Geometry: final body of the model. Coordinates: model frame, mm. A direction names the side the tool comes from. Give positions to 0.01 mm unless a question says otherwise; leave off trailing zeros. Write each loop counter-clockwise with the first axis right and the second up, starting at its lowest first coordinate (ties: lowest second). Pieces come first, ordered by that corner, then holes. Notation, with made-up numbers: M 41,27.5 L 48,27.5 A22 cw 48,66.5 Z; hole C 75,1.5 d9. An arc over 180 degrees is marked long. Answer as a JSON object with one key per item and string values.
from build123d import *

# Parameters (mm, degrees)
F0_R          = 342.9
F0_R_2        = 303.53
F1_DEPTH      = 91.44
F1_DEPTH_BACK = 36
F2_R          = 307.34
F2_R_2        = 303.53
F3_DEPTH      = 60.96
F4_R          = 307.34
F4_R_2        = 303.53
F5_DEPTH      = 24


with BuildPart() as f1:
    # F0 (on Front) → F1 (new body, two sides)
    with BuildSketch(Plane.XZ) as f1_sk:
        Circle(F0_R)
        Circle(F0_R_2, mode=Mode.SUBTRACT)
    extrude(amount=F1_DEPTH)
    extrude(f1_sk.sketch, amount=-F1_DEPTH_BACK)

    # F2 (on face) → F3 (cut)
    with BuildSketch(Plane.XZ.offset(91.44)):
        Circle(F2_R)
        Circle(F2_R_2, mode=Mode.SUBTRACT)
    extrude(amount=-F3_DEPTH, mode=Mode.SUBTRACT)

    # F4 (on face) → F5 (cut)
    with BuildSketch(Plane(origin=(0, 36, 0), x_dir=(-1, 0, 0), z_dir=(0, 1, 0))):
        Circle(F4_R)
        Circle(F4_R_2, mode=Mode.SUBTRACT)
    extrude(amount=-F5_DEPTH, mode=Mode.SUBTRACT)


solid = f1.part
1) Cut plane C-C on y = -42. Return loops of the section in (x, z).
Geometry check:
{"outline": "C 0,0 d685.8; hole C 0,0 d614.68"}
2) Cut plane A-A on x = 0. Return loops of the section in (y, z), and give its area (3 significant figures).
Geometry check:
{"outline": "M -91.44,-342.9 L 36,-342.9 L 36,-307.34 L 12,-307.34 L 12,-303.53 L -30.48,-303.53 L -30.48,-307.34 L -91.44,-307.34 Z; M -91.44,307.34 L -30.48,307.34 L -30.48,303.53 L 12,303.53 L 12,307.34 L 36,307.34 L 36,342.9 L -91.44,342.9 Z", "area": "9,390 mm2"}
3) Line query: line 1 (Z direction, x = 0, y = -54); line 2 (Z direction, x = 0, y = -2); line 3 (Z direction, x = -312, y = -42). Output: solid intervals per line, ascending. Write a range as from..to.
Geometry check:
{"line 1": "z = -342.9..-307.34, 307.34..342.9", "line 2": "z = -342.9..-303.53, 303.53..342.9", "line 3": "z = -142.25..142.25"}
4) Contact query for flat-ended pins moving along their axis: P1, Ø5, axis at x = 205, y = -68.5, coming from the +Z side; P2, Ø8, axis at y = -19, z = 263, coming from the +X side; P3, Ø3, axis at x = -168, y = -66, coming from the -Z side. Output: stop coordinate, or through.
Geometry check:
{"P1": "stops at z = 276.72", "P2": "stops at x = 224.72", "P3": "stops at z = -299.76"}
5) Set-up query: faces 1 (the flat face through (70, 12, 297)), 2 (the cylindrical face through (293.148, -61.387, 92.317)), 3 (the flat face through (-129, 36, 281)). Return all of +Z, -Z, +X, -X, +Y, -Y with unobstructed straight access to the full face (end or side cutting, diameter ignored); none if empty.
Geometry check:
{"face 1": "+Y", "face 2": "-Y", "face 3": "+Z, -Z, +X, -X, +Y"}
6) Cut plane B-B on z = 0. Return loops of the section in (x, y), and give its area (3 significant figures).
Geometry check:
{"outline": "M -342.9,-91.44 L -307.34,-91.44 L -307.34,-30.48 L -303.53,-30.48 L -303.53,12 L -307.34,12 L -307.34,36 L -342.9,36 Z; M 303.53,-30.48 L 307.34,-30.48 L 307.34,-91.44 L 342.9,-91.44 L 342.9,36 L 307.34,36 L 307.34,12 L 303.53,12 Z", "area": "9,390 mm2"}
7) Pull-direction query (Z, two-part tool) for faces 4 (the flat face through (-70, -30.48, 297)), 5 (the flat face through (-129, -91.44, 281)), 6 (the cylindrical face through (184.341, -28.612, 289.135)), 7 (the cylindrical face through (-223.714, -9.537, 205.14)); classes: pulls with the +Z half, pulls with the -Z half, needs draft (parallel to the pull), parting line crosses it, or undercut.
Geometry check:
{"face 4": "undercut", "face 5": "needs draft", "face 6": "parting line crosses it", "face 7": "undercut"}
